from build123d import *

# Parameters (mm, degrees)
F3_R      = 6.35
F4_DEPTH  = 63.5
F3_R_2    = 12.7
F5_DEPTH  = 50.8
F3_R_3    = 19.05
F6_DEPTH  = 38.1
F3_R_4    = 25.4
F7_DEPTH  = 25.4
F3_R_5    = 31.75
F8_DEPTH  = 12.7
F10_R     = 9.525
F11_DEPTH = 12.7
F14_R     = 1.27


# Not quite as in the source:
# - a fillet or chamfer that OpenCascade refuses, or shapes differently, is made with other operations: its cross-section is extruded or revolved along the edge and cut away or added


with BuildPart() as f1:
    # F0 (on Top) → F1 (revolve)
    with BuildSketch(Plane.XY):
        with BuildLine():
            ThreePointArc((0, -38.1), (26.9407683632, -26.9407683632), (38.1, 0))
            ThreePointArc((38.1, 0), (26.9407683632, 26.9407683632), (0, 38.1))
            Line((0, 38.1), (0, -38.1))
        make_face()
    revolve(axis=Axis((0, 0, 0), (0, 1, 0)))

    # F3 (on offset) → F4 (cut)
    with BuildSketch(Plane.XZ.offset(38.1)):
        Circle(F3_R)
    extrude(amount=-F4_DEPTH, mode=Mode.SUBTRACT)

    # F3 (on offset) → F5 (cut)
    with BuildSketch(Plane.XZ.offset(38.1)):
        Circle(F3_R_2)
        Circle(F3_R, mode=Mode.SUBTRACT)
    extrude(amount=-F5_DEPTH, mode=Mode.SUBTRACT)

    # F3 (on offset) → F6 (cut)
    with BuildSketch(Plane.XZ.offset(38.1)):
        Circle(F3_R_3)
        Circle(F3_R_2, mode=Mode.SUBTRACT)
    extrude(amount=-F6_DEPTH, mode=Mode.SUBTRACT)

    # F3 (on offset) → F7 (cut)
    with BuildSketch(Plane.XZ.offset(38.1)):
        Circle(F3_R_4)
        Circle(F3_R_3, mode=Mode.SUBTRACT)
    extrude(amount=-F7_DEPTH, mode=Mode.SUBTRACT)

    # F3 (on offset) → F8 (cut)
    with BuildSketch(Plane.XZ.offset(38.1)):
        Circle(F3_R_5)
        Circle(F3_R_4, mode=Mode.SUBTRACT)
    extrude(amount=-F8_DEPTH, mode=Mode.SUBTRACT)

    # F10 (on offset) → F11 (join, symmetric)
    with BuildSketch(Plane.XY.offset(38.1)):
        Circle(F10_R)
    extrude(amount=F11_DEPTH, both=True)

    # F12: fillet of radius 7.62 on 1 edges, made by hand

    # F12_s1 → F12_t2 (revolve)
    with BuildSketch(Plane.XZ):
        with BuildLine():
            ThreePointArc((14.2875000004, 35.3196452948), (10.8268297748, 38.1238648566), (9.5250000004, 42.3835743538))
            Line((9.5250000004, 42.3835743538), (9.525, 36.8901663726))
            ThreePointArc((9.525, 36.8901663726), (11.9321172967, 36.1833466781), (14.2875000004, 35.3196452948))
        make_face()
    revolve(axis=Axis((2e-10, 0, 36.8901663726), (0, 0, 1)))

    # F15: sweep along a path in F13
    with BuildLine(Plane.XZ) as f15_path:
        ThreePointArc((6.35, 50.8), (0, 57.15), (-6.35, 50.8))
    # F14 (on face) → F15 (sweep)
    with BuildSketch(Plane.XY.offset(50.8)):
        with Locations((-6.35, 0)):
            Circle(F14_R)
    sweep(path=f15_path.line)


solid = f1.part
Build history of the part. All positions in model axes, mm. A direction names the side the tool comes from. Give positions to 0.01 mm unless a question says otherwise; leave off trailing zeros. Loops run counter-clockwise (first coordinate to the right, second up) from the corner with the lowest first, then second, coordinate; pieces in that order, holes last. Notation, with made-up numbers: (77.25, -8) - (101.25, -8) arc R23 ccw to (101.25, 30) - close; hole circle Ø1 at (39.5, 75.25). An arc over 180 degrees is marked (long way). Write item = value, one per line. Start each with the question number.
1) Tool access for faces 1 (the flat face through (-21, -25.4, -15)), 2 (the cylindrical face through (-5.506, -19.139, -24.796)): list every direction of +Z, -Z, +X, -X, +Y, -Y with a clear straight run to the whole face (end or side of a thin tool).
2) Pull direction Z, two halves, no side cores. Call faces 3 (the cylindrical face through (-1.38, 18.96, -6.2)), 4 (the cylindrical face through (-7.559, -5.796, 46.651)): +Z half, -Z half, draft (parallel to the pull), parting line (faces both ways), or undercut.
3) Probe probe 1 along Z at (x, y) = (0, -19); probe 2 along Z at (x, y) = (0, -22); probe 3 along X at (y, z) = (17, -25). List the from-to ranges inside material, lowest first. Write a range as from..to.
4) Drop flat-ended pins along their axis: pin 1 Ø1.5 at (y, z) = (-3.5, -15) entering from +X; pin 2 Ø1 at (x, z) = (5.5, 7.5) entering from +Y; pin 3 Ø15 at (x, z) = (-10.5, 9.5) entering from -Y; pin 4 Ø9.5 at (x, y) = (-1.5, 1) entering from +Z. Give the stop position or say it passes through.
5) Band-saw the part on D-D on z = 14.5. Give the cut face in (x, y), plus the area to 3 significant figures.
6) Band-saw the part on B-B on y = 15.5. Give the cut face in (x, z).
7) Band-saw the part on C-C on x = 17. Give the cut face in (y, z).
8) Band-saw the part on A-A on z = 0. Give the cut face in (x, y).
Final values:
q1.face_1 = +Z, -Z, +X, -X, -Y
q1.face_2 = -Y
q2.face_3 = undercut
q2.face_4 = draft
q3.probe_1 = -33.02..-25.4, 25.4..33.02
q3.probe_2 = -31.11..-25.4, 25.4..31.11
q3.probe_3 = -23.19..23.19
q4.pin_1 = 35.17
q4.pin_2 = 37.07
q4.pin_3 = -12.7
q4.pin_4 = 58.42
q5.outline = (-24.42, -25.4) - (-20.85, -25.4) - (-20.85, -12.7) - (-12.36, -12.7) - (-12.36, 0) - (12.36, 0) - (12.36, -12.7) - (20.85, -12.7) - (20.85, -25.4) - (24.42, -25.4) arc R35.23 ccw (long way) to start
q5.area = 2,730 mm²
q6.outline = circle Ø69.61 at (0, 0); hole circle Ø12.7 at (0, 0)
q7.outline = (-25.4, -22.75) arc R34.1 ccw (long way) to (-25.4, 22.75) - (-25.4, 18.87) - (-12.7, 18.87) - (-12.7, 8.6) - (0, 8.6) - (0, -8.6) - (-12.7, -8.6) - (-12.7, -18.87) - (-25.4, -18.87) - close
q8.outline = (-28.4, -25.4) - (-25.4, -25.4) - (-25.4, -12.7) - (-19.05, -12.7) - (-19.05, 0) - (-12.7, 0) - (-12.7, 12.7) - (-6.35, 12.7) - (-6.35, 25.4) - (6.35, 25.4) - (6.35, 12.7) - (12.7, 12.7) - (12.7, 0) - (19.05, 0) - (19.05, -12.7) - (25.4, -12.7) - (25.4, -25.4) - (28.4, -25.4) arc R38.1 ccw (long way) to start
